Can you work these out from the model? Positions are in its coordinate system, mm. A direction names the side the tool comes from. Give positions to 0.01 mm unless a question says otherwise; leave off trailing zeros. Loops run counter-clockwise (first coordinate to the right, second up) from the corner with the lowest first, then second, coordinate; pieces in that order, holes last. Notation, with made-up numbers: (11, 50.5) - (57, 50.5) arc R28 cw to (57, 69.5) - close; hole circle Ø1 at (-6, 10). An arc over 180 degrees is marked (long way). Answer in a Markdown table with one row per item.
from build123d import *

# Parameters (mm, degrees)
SKETCH9_R      = 3.175
SKETCH9_R_2    = 2.413
EXTRUDE1_DEPTH = 1.016


with BuildPart() as part:
    # Sketch8 → Revolve1 (revolve)
    with BuildSketch(Plane(origin=(0, 0, 0), x_dir=(0, 0, -1), z_dir=(1, 0, 0)), mode=Mode.PRIVATE) as revolve1_sk:
        with BuildLine():
            Line((13.335, 4.9149), (13.97, 4.9149))
            ThreePointArc((13.97, 4.9149), (14.508815367, 4.691715367), (14.732, 4.1529))
            Line((14.732, 4.1529), (14.732, 3.556))
            Line((14.732, 3.556), (14.351, 3.175))
            Line((14.351, 3.175), (0, 3.175))
            Line((0, 3.175), (0, 4.3688))
            Line((0, 4.3688), (1.636888889, 4.3688))
            Line((1.636888889, 4.3688), (3.528634781, 5.461))
            Line((3.528634781, 5.461), (12.319, 5.461))
            Line((12.319, 5.461), (12.319, 4.42341))
            Line((12.319, 4.42341), (13.335, 4.42341))
            Line((13.335, 4.42341), (13.335, 4.9149))
        make_face()
    revolve1 = revolve(revolve1_sk.sketch.rotate(Axis((0, 0, 0), (0, 0, -1)), 90), axis=Axis((0, 0, 0), (0, 0, -1)))  # turned: the seam where the file's is

    # Sketch9 → Extrude1 (add)
    with BuildSketch(Plane.XY):
        Circle(SKETCH9_R)
        Circle(SKETCH9_R_2, mode=Mode.SUBTRACT)
    extrude(amount=-EXTRUDE1_DEPTH)

    # Mirror1: Revolve1 across plane
    add(revolve1.mirror(Plane.XY))


solid = part.part
Q1. If I drill on line 1 (Y direction, x = 0, z = 5) (3 decimals); line 2 (Y direction, x = 0, z = -0.3); line 3 (Z direction, x = 4, y = 2.5) (3 decimals), over which ranges is the centre line in solid material (lowest first)? Write a range as [from, to].
Checked values:
| item | result |
|---|---|
| line 1 | y = [-5.461, -3.175], [3.175, 5.461] |
| line 2 | y = [-4.37, -2.41], [2.41, 4.37] |
| line 3 | z = [-14.482, -13.335], [-12.319, -2.24], [2.24, 12.319], [13.335, 14.482] |
Q2. If we mould it in two halves opening along X, with no side actions, what happens to faces 4 (the face through (-1.915, -1.468, -0.501)), 5 (the face through (5.21, -1.64, -7.99))? For each: released by +X, released by -X, zero draft, split by the parting line, or undercut.
Checked values:
| item | result |
|---|---|
| face 4 | undercut |
| face 5 | split by the parting line |
Q3. For pin 1 (3 mm diameter, centred on x = -1, y = -0.5, fed in from +Z); pin 2 (4 mm diameter, centred on x = 3.5, z = -5.5, fed in from -Y); pin 3 (4 mm diameter, centred on x = 2.5, z = 8, fed in from +Y), each with a flat end and sliding along its axis, tell me the tip position at first contact or that it passes through.
Checked values:
| item | result |
|---|---|
| pin 1 | stops at z = 0 |
| pin 2 | stops at y = -5.25 |
| pin 3 | stops at y = 5.44 |
Q4. On a 3-axis mill with a long thin cutter (end or side, diameter ignored), from which of +Z, -Z, +X, -X, +Y, -Y can I reach the whole of each face in a straight line? I mean faces 1 (the face through (4.167, -1.312, 0.023)), 2 (the face through (2.27, 4.36, 13.66)), 3 (the face through (-2.52, 1.93, -7.59)). Say none if no direction works.
Checked values:
| item | result |
|---|---|
| face 1 | none |
| face 2 | +Z |
| face 3 | -Z |
Q5. Imagine slicing it at A-A, the plane z = -5.25. Write out the boundary of the cut face in (x, y) (3 decimals), and give its area (3 significant figures).
Checked values:
| item | result |
|---|---|
| outline | circle Ø10.922 at (0, 0); hole circle Ø6.35 at (0, 0) |
| area | 62.0 mm² |
